Source: CAD feature listing. Evaluate the final solid. Frame: model axes, mm. Face numbers are marked on the shaded views. A direction names the side the tool comes from. Give positions to 0.01 mm unless a question says otherwise; leave off trailing zeros. Write each loop counter-clockwise with the first axis right and the second up, starting at its lowest first coordinate (ties: lowest second). Pieces come first, ordered by that corner, then holes. Notation, with made-up numbers: M -36,17.25 L -23,17.25 A27 cw -23,36.25 Z; hole C 13.25,56.25 d11. An arc over 180 degrees is marked long. Answer as a JSON object with one key per item and string values. Group by question number.
```python
from build123d import *

# Parameters (mm, degrees)
F1_DEPTH = 16
F2_R     = 6.5
F3_DEPTH = 93.001
F4_DEPTH = 93.001


with BuildPart() as f1:
    # F0 (on Front) → F1 (new body, symmetric)
    with BuildSketch(Plane.XZ):
        Polygon((0, 13), (0, 0), (39, 0), (39, 13), (74, 13), (74, 0), (113, 0), (113, 13), (93, 13), (93, 64), (74, 64), (74, 26), (39, 26), (39, 64), (20, 64), (20, 13), align=None)
    extrude(amount=F1_DEPTH, both=True)

    # F2 (on face) → F3 (cut, through all)
    with BuildSketch(Plane.YZ.offset(93)):
        with Locations((0, 46)):
            Circle(F2_R)
    extrude(amount=-F3_DEPTH, mode=Mode.SUBTRACT)

    # F2 (on face) → F4 (cut, through all)
    with BuildSketch(Plane.YZ.offset(93)):
        with Locations((0, 46)):
            Circle(F2_R)
    extrude(amount=-F4_DEPTH, mode=Mode.SUBTRACT)


solid = f1.part
```
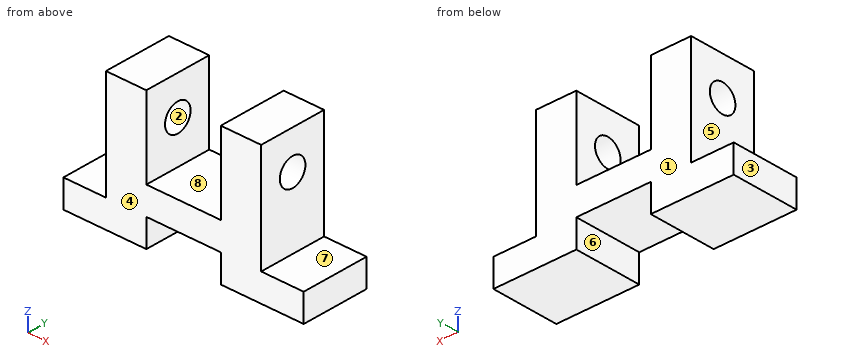
(1) Pull-direction query (Y, two-part tool) for the marked faces 1, 2, 3 and 4; classes: pulls with the +Y half, pulls with the -Y half, needs draft (parallel to the pull), parting line crosses it, or undercut.
(2) Access query for the marked faces 5, 6, 7 and 8. Directions: +Z, -Z, +X, -X, +Y, -Y. A direction counts if a zero-diameter tool reaches every point of the face in a straight line with its end or side. Return the directions, or none.
(3) Section C-C, the plane z = 46. Return loops of the section in (x, y), plus the area to 3 significant figures.
(4) Section B-B, the plane z = 5. Return loops of the section in (x, y), plus the area to 3 significant figures.
(5) Ray query, L1, parallel to X at y = -4, z = 55; L2, parallel to X at y = -8.5, z = 4.5; L3, parallel to Z at x = 25.5, y = 0. Return the intervals inside material, ascending. Write a range as [from, to].
(6) Contact query for flat-ended pins moving along their axis: pin 1 Ø9.5 at (x, y) = (59.5, 5.5) entering from -Z; pin 2 Ø10 at (x, y) = (103.5, 2.5) entering from +Z; pin 3 Ø1.5 at (y, z) = (-8.5, 46) entering from +X; pin 4 Ø16 at (x, y) = (14, -5.5) entering from +Z. Output: stop coordinate, or through.
(7) Section D-D, the plane x = 81.5. Return loops of the section in (y, z).
(8) Section A-A, the plane y = 0. Return loops of the section in (x, z).
Reported:
{
 "1": {"face 1": "pulls with the +Y half", "face 2": "undercut", "face 3": "needs draft", "face 4": "pulls with the -Y half"},
 "2": {"face 5": "+Z, -X, +Y, -Y", "face 6": "-Z, +Y, -Y", "face 7": "+Z, +X, +Y, -Y", "face 8": "+Z, +Y, -Y"},
 "3": {"outline": "M 20,-16 L 39,-16 L 39,-6.5 L 20,-6.5 Z; M 20,6.5 L 39,6.5 L 39,16 L 20,16 Z; M 74,-16 L 93,-16 L 93,-6.5 L 74,-6.5 Z; M 74,6.5 L 93,6.5 L 93,16 L 74,16 Z", "area": "722 mm2"},
 "4": {"outline": "M 0,-16 L 39,-16 L 39,16 L 0,16 Z; M 74,-16 L 113,-16 L 113,16 L 74,16 Z", "area": "2,500 mm2"},
 "5": {"L1": "x = [20, 39], [74, 93]", "L2": "x = [0, 39], [74, 113]", "L3": "z = [0, 39.5], [52.5, 64]"},
 "6": {"pin 1": "stops at z = 13", "pin 2": "stops at z = 13", "pin 3": "stops at x = 93", "pin 4": "stops at z = 64"},
 "7": {"outline": "M -16,0 L 16,0 L 16,64 L -16,64 Z; hole C 0,46 d13"},
 "8": {"outline": "M 0,0 L 39,0 L 39,13 L 74,13 L 74,0 L 113,0 L 113,13 L 93,13 L 93,39.5 L 74,39.5 L 74,26 L 39,26 L 39,39.5 L 20,39.5 L 20,13 L 0,13 Z; M 20,52.5 L 39,52.5 L 39,64 L 20,64 Z; M 74,52.5 L 93,52.5 L 93,64 L 74,64 Z"}
}
